```python
from build123d import *

# Parameters (mm, degrees)
CYLINDER1697_R              = 1.5
CYLINDER1697_DEPTH          = 20
CYLINDER1698_R              = 1.5
CYLINDER1698_DEPTH          = 20
COMPOUND842_ROLL_ANGLE      = 90
COMPOUND842_PLACEMENT_ANGLE = 90
CYLINDER1690_R              = 2.5
CYLINDER1690_DEPTH          = 20
CYLINDER1689_R              = 2.5
CYLINDER1689_DEPTH          = 20
CYLINDER1696_R              = 5
CYLINDER1696_DEPTH          = 5
CYLINDER1687_R              = 5
CYLINDER1687_DEPTH          = 5
CYLINDER1695_R              = 3
CYLINDER1695_DEPTH          = 3
CYLINDER1692_R              = 3
CYLINDER1692_DEPTH          = 3
CYLINDER1693_R              = 3
CYLINDER1693_DEPTH          = 3
CYLINDER1694_R              = 3
CYLINDER1694_DEPTH          = 3
CYLINDER1682_R              = 1.5
CYLINDER1682_DEPTH          = 60
CYLINDER1685_R              = 1.5
CYLINDER1685_DEPTH          = 60
CYLINDER1683_R              = 1.5
CYLINDER1683_DEPTH          = 60
CYLINDER1681_R              = 1.5
CYLINDER1681_DEPTH          = 60
CYLINDER1677_R              = 5
CYLINDER1677_DEPTH          = 5
BOX657_W                    = 104
BOX657_H                    = 20
BOX657_DEPTH                = 4
CHAMFER049_SIZE             = 4
CHAMFER050_SIZE             = 2


with BuildPart() as obj1:
    # Cylinder1697 → Cylinder1697 (new body)
    with BuildSketch(Plane(origin=(15.75, 114, 58.525), x_dir=(-1, 0, 0), z_dir=(0, 1, 0))):
        Circle(CYLINDER1697_R)
    extrude(amount=CYLINDER1697_DEPTH)


with BuildPart() as compound840:
    # Cylinder1698 → Cylinder1698 (new body)
    with BuildSketch(Plane(origin=(15.75, 114, 39.475), x_dir=(-1, 0, 0), z_dir=(0, 1, 0))):
        Circle(CYLINDER1698_R)
    extrude(amount=CYLINDER1698_DEPTH)

    # Compound842: union obj1
    add(obj1.part)


with BuildPart() as compound840_1:
    # Compound842 roll: moved
    add(compound840.part.rotate(Axis((0, 0, 0), (1, 0, 0)), COMPOUND842_ROLL_ANGLE))


with BuildPart() as compound840_2:
    # Compound842 placement: moved
    add(compound840_1.part.moved(Location((-49, 0, -96))).rotate(Axis((-49, 0, -96), (0, 0, 1)), COMPOUND842_PLACEMENT_ANGLE))


with BuildPart() as compound840_3:
    # Compound840 placement: moved
    add(compound840_2.part.moved(Location((0, 74, -72))))


with BuildPart() as obj2:
    # Cylinder1690 → Cylinder1690 (new body)
    with BuildSketch(Plane(origin=(-42, 90, -59), x_dir=(1, 0, 0), z_dir=(0, 0, 1))):
        Circle(CYLINDER1690_R)
    extrude(amount=CYLINDER1690_DEPTH)


with BuildPart() as compound837:
    # Cylinder1689 → Cylinder1689 (new body)
    with BuildSketch(Plane(origin=(42, 90, -59), x_dir=(1, 0, 0), z_dir=(0, 0, 1))):
        Circle(CYLINDER1689_R)
    extrude(amount=CYLINDER1689_DEPTH)

    # Compound837: union obj2
    add(obj2.part)


with BuildPart() as obj3:
    # Cylinder1696 → Cylinder1696 (new body)
    with BuildSketch(Plane(origin=(-42, 90, -59), x_dir=(1, 0, 0), z_dir=(0, 0, 1))):
        Circle(CYLINDER1696_R)
    extrude(amount=CYLINDER1696_DEPTH)


with BuildPart() as compound836:
    # Cylinder1687 → Cylinder1687 (new body)
    with BuildSketch(Plane(origin=(42, 90, -59), x_dir=(1, 0, 0), z_dir=(0, 0, 1))):
        Circle(CYLINDER1687_R)
    extrude(amount=CYLINDER1687_DEPTH)

    # Compound836: union obj3
    add(obj3.part)


with BuildPart() as obj4:
    # Cylinder1695 → Cylinder1695 (new body)
    with BuildSketch(Plane(origin=(18, 85, -57), x_dir=(1, 0, 0), z_dir=(0, 0, 1))):
        Circle(CYLINDER1695_R)
    extrude(amount=CYLINDER1695_DEPTH)


with BuildPart() as obj5:
    # Cylinder1692 → Cylinder1692 (new body)
    with BuildSketch(Plane(origin=(-18, 85, -57), x_dir=(1, 0, 0), z_dir=(0, 0, 1))):
        Circle(CYLINDER1692_R)
    extrude(amount=CYLINDER1692_DEPTH)


with BuildPart() as obj6:
    # Cylinder1693 → Cylinder1693 (new body)
    with BuildSketch(Plane(origin=(-18, 95, -57), x_dir=(1, 0, 0), z_dir=(0, 0, 1))):
        Circle(CYLINDER1693_R)
    extrude(amount=CYLINDER1693_DEPTH)


with BuildPart() as compound834:
    # Cylinder1694 → Cylinder1694 (new body)
    with BuildSketch(Plane(origin=(18, 95, -57), x_dir=(1, 0, 0), z_dir=(0, 0, 1))):
        Circle(CYLINDER1694_R)
    extrude(amount=CYLINDER1694_DEPTH)

    # Compound834: union obj4, obj5, obj6
    add(obj4.part)
    add(obj5.part)
    add(obj6.part)


with BuildPart() as obj7:
    # Cylinder1682 → Cylinder1682 (new body)
    with BuildSketch(Plane(origin=(18, 85, -57), x_dir=(1, 0, 0), z_dir=(0, 0, 1))):
        Circle(CYLINDER1682_R)
    extrude(amount=CYLINDER1682_DEPTH)


with BuildPart() as obj8:
    # Cylinder1685 → Cylinder1685 (new body)
    with BuildSketch(Plane(origin=(-18, 85, -57), x_dir=(1, 0, 0), z_dir=(0, 0, 1))):
        Circle(CYLINDER1685_R)
    extrude(amount=CYLINDER1685_DEPTH)


with BuildPart() as obj9:
    # Cylinder1683 → Cylinder1683 (new body)
    with BuildSketch(Plane(origin=(-18, 95, -57), x_dir=(1, 0, 0), z_dir=(0, 0, 1))):
        Circle(CYLINDER1683_R)
    extrude(amount=CYLINDER1683_DEPTH)


with BuildPart() as compound833:
    # Cylinder1681 → Cylinder1681 (new body)
    with BuildSketch(Plane(origin=(18, 95, -57), x_dir=(1, 0, 0), z_dir=(0, 0, 1))):
        Circle(CYLINDER1681_R)
    extrude(amount=CYLINDER1681_DEPTH)

    # Compound833: union obj7, obj8, obj9
    add(obj7.part)
    add(obj8.part)
    add(obj9.part)


with BuildPart() as obj10:
    # Cylinder1677 → Cylinder1677 (new body)
    with BuildSketch(Plane(origin=(0, 90, -54), x_dir=(1, 0, 0), z_dir=(0, 0, 1))):
        Circle(CYLINDER1677_R)
    extrude(amount=CYLINDER1677_DEPTH)


with BuildPart() as cut344:
    # Box657 → Box657 (new body)
    with BuildSketch(Plane(origin=(-52, 80, -56), x_dir=(1, 0, 0), z_dir=(0, 0, 1))):
        with Locations((52, 10)):
            Rectangle(BOX657_W, BOX657_H)
    extrude(amount=BOX657_DEPTH)

    # Cut337: cut obj10
    add(obj10.part, mode=Mode.SUBTRACT)

    # Cut339: cut Compound833
    add(compound833.part, mode=Mode.SUBTRACT)

    # Cut340: cut Compound834
    add(compound834.part, mode=Mode.SUBTRACT)

    # Cut338: cut Compound836
    add(compound836.part, mode=Mode.SUBTRACT)

    # Cut341: cut Compound837
    add(compound837.part, mode=Mode.SUBTRACT)

    # Chamfer049
    chamfer049_edges = [cut344.edges().sort_by_distance(p)[0] for p in [
        (-52, 100, -54),
        (52, 100, -54),
    ]]
    chamfer(chamfer049_edges, length=CHAMFER049_SIZE)

    # Chamfer050
    chamfer050_edges = [cut344.edges().sort_by_distance(p)[0] for p in [
        (-52, 88, -56),
        (52, 88, -56),
    ]]
    chamfer(chamfer050_edges, length=CHAMFER050_SIZE)

    # Cut344: cut Compound840
    add(compound840_3.part, mode=Mode.SUBTRACT)


solid = cut344.part
```
Check sheet for the modelled part. Datum: model origin and axes. Units: mm. A direction names the side the tool comes from. Round coordinates to 2 decimals unless told otherwise and drop trailing zeros. Order: outer loops, then holes, each group sorted by start corner. A loop starts at its lowest first (then second) coordinate and runs counter-clockwise, first axis right, second up. Notation, with made-up numbers: (44.5, 28) -> (86.5, 28) arc R14 cw to (86.5, 38) -> close; hole circle Ø3 at (-38, 45). An arc over 180 degrees is marked (long way). One line per item, written item: value. Start each with the question number.
Q1. Cross-section at A-A (x = -18). Record the boundary of the cut face in (y, z), and give its area (3 significant figures).
Q2. Cross-section at C-C (z = -55.1). Record the boundary of the cut face in (x, y).
Q3. Thickness scan on line 1 (Y direction, x = 18, z = -53.3); line 2 (Y direction, x = -18, z = -55.1); line 3 (X direction, y = 87.75, z = -55). Record the ranges inside material, lowest first.
Q4. Cross-section at D-D (y = 90). Give the number of separate pieces and of enclosed holes in the cut face, and give its area (3 significant figures).
Q5. Cross-section at B-B (x = -42). Record the boundary of the cut face in (y, z).
Q6. Set-up check for faces 1 (the face through (-1.08, 85.12, -53.01)), 2 (the face through (-18.65, 82.07, -55.01)), 3 (the face through (41.67, 92.48, -53.01)): record each of +Z, -Z, +X, -X, +Y, -Y from which the full face is reachable in a straight line by a thin tool's end or side.
Q7. Mould release check, pull along Y, two halves, no side actions. Record for faces 4 (the face through (52, 88, -53)), 5 (the face through (-1, 80, -54)), 6 (the face through (-1, 100, -54)), 7 (the face through (-40, 88, -54)): pulls with the +Y half, pulls with the -Y half, needs draft (parallel to the pull), parting line crosses it, or undercut.
Q8. Gauge pin test, flat ends, axial feed: pin 1 Ø3.5 at (x, y) = (-18, 95) entering from -Z; pin 2 Ø5 at (x, y) = (16.5, 94.5) entering from -Z; pin 3 Ø0.9 at (x, y) = (-9.5, 89.5) entering from +Z. Record the tip position at first contact, or that the pin passes through.
Completed:
1. outline: (80, -56) -> (82, -56) -> (82, -54) -> (83.5, -54) -> (83.5, -52) -> (80, -52) -> close; (86.5, -54) -> (88, -54) -> (88, -56) -> (92, -56) -> (92, -54) -> (93.5, -54) -> (93.5, -52) -> (86.5, -52) -> close; (96.5, -54) -> (98, -54) -> (98, -56) -> (100, -56) -> (100, -52) -> (96.5, -52) -> close
1. area: 44.0 mm²
2. outline: (-50.9, 80) -> (50.9, 80) -> (50.9, 97.1) -> (48, 100) -> (-48, 100) -> (-50.9, 97.1) -> close; hole circle Ø10 at (-42, 90); hole circle Ø6 at (-18, 85); hole circle Ø6 at (-18, 95); hole circle Ø6 at (18, 85); hole circle Ø6 at (18, 95); hole circle Ø10 at (42, 90)
3. line 1: y = 80 to 83.5, 86.5 to 93.5, 96.5 to 100
3. line 2: y = 80 to 82, 88 to 92, 98 to 100
3. line 3: x = -51 to -46.47, -37.53 to -19.2, -16.8 to 16.8, 19.2 to 37.53, 46.47 to 51
4. separate pieces: 3
4. enclosed holes: 0
4. area: 320 mm²
5. outline: (80, -56) -> (85, -56) -> (85, -54) -> (87.5, -54) -> (87.5, -52) -> (80, -52) -> close; (92.5, -54) -> (95, -54) -> (95, -56) -> (100, -56) -> (100, -52) -> (92.5, -52) -> close
6. face 1: +Z
6. face 2: -Z
6. face 3: +Z, -Z
7. face 4: needs draft
7. face 5: pulls with the -Y half
7. face 6: pulls with the +Y half
7. face 7: undercut
8. pin 1: stops at z = -54
8. pin 2: stops at z = -56
8. pin 3: stops at z = -54
